from build123d import *

# Parameters (mm, degrees)
CHAMFER1_SIZE = 1
CHAMFER2_SIZE = 0.2


with BuildPart() as part:
    # Sketch1 → Revolve1 (revolve)
    with BuildSketch(Plane(origin=(0, 0, 0), x_dir=(0, 0, -1), z_dir=(1, 0, 0))):
        Polygon((4.1, 18), (21, 18), (21, 14), (12, 14), (12, 6.35), (6.8, 6.35), (6.8, -6.35), (12, -6.35), (12, -14), (21, -14), (21, -18), (4.1, -18), align=None)
    revolve(axis=Axis((0, -56.19047619, 0), (0, 1, 0)))

    # Chamfer1
    chamfer1_edges = [part.edges().sort_by_distance(p)[0] for p in [
        (0, -14, 21),
        (0, 14, 21),
        (0, 6.35, 12),
        (0, -6.35, 12),
    ]]
    chamfer(chamfer1_edges, length=CHAMFER1_SIZE)

    # Chamfer2
    chamfer2_edges = [part.edges().sort_by_distance(p)[0] for p in [
        (0, 14, 12),
        (0, 6.35, 6.8),
        (0, -6.35, 6.8),
        (0, -14, 12),
    ]]
    chamfer(chamfer2_edges, length=CHAMFER2_SIZE)


solid = part.part
Model file for the job. Use its own axes, mm. A direction names the side the tool comes from. Round coordinates to 2 decimals unless told otherwise and drop trailing zeros. Order: outer loops, then holes, each group sorted by start corner. A loop starts at its lowest first (then second) coordinate and runs counter-clockwise, first axis right, second up.
(1) Pull direction Z, two halves, no side cores. Call faces 3 (the face through (-6.31, 16.48, -20.03)), 4 (the face through (-4.065, 0.252, 0.534)), 5 (the face through (-9, -14, 9)): released by +Z, released by -Z, zero draft, split by the parting line, or undercut.
(2) 3-axis set-ups, long thin cutter, end or side, ignore diameter. For faces 1 (the face through (-0.53, -10.62, 11.99)), 2 (the face through (-0.3, -18, -4.4)): which of +Z, -Z, +X, -X, +Y, -Y reach the whole face in a straight line?
(3) Pin check, flat tips, straight feed: pin 1 (10 mm diameter, centred on x = 15.5, y = 0.5, fed in from -Z); pin 2 (9.5 mm diameter, centred on x = 0, z = 0, fed in from +Y); pin 3 (12 mm diameter, centred on y = -10, z = -14, fed in from -X); pin 4 (12 mm diameter, centred on x = 11, y = -4.5, fed in from +Z). Stop position of each tip, or through.
(4) Band-saw the part on A-A (y = 0). List the corners of the cut face in (x, z), then the cut area to 3 significant figures.
(5) Band-saw the part on B-B (y = -8.5). List the corners of the cut face in (x, z), then the cut area to 3 significant figures.
(6) Drill centre lines: line 1 (X direction, y = -5, z = 0); line 2 (Y direction, x = -1.5, z = 13.5). Where is each one in solid material? Low to high.
Verdict:
1. face 3: split by the parting line
1. face 4: undercut
1. face 5: zero draft
2. face 1: none
2. face 2: +Z, -Z, +X, -X, -Y
3. pin 1: passes through
3. pin 2: stops at y = 18
3. pin 3: stops at x = -18.08
3. pin 4: stops at z = 10.55
4. outline: circle Ø13.6 at (0, 0); hole circle Ø8.2 at (0, 0)
4. area: 92.5 mm2
5. outline: circle Ø24 at (0, 0); hole circle Ø8.2 at (0, 0)
5. area: 400 mm2
6. line 1: x = -6.8 to -4.1, 4.1 to 6.8
6. line 2: y = -18 to -14, 14 to 18
